Source: CAD feature listing. Evaluate the final solid. Frame: model axes, mm. A direction names the side the tool comes from. Give positions to 0.01 mm unless a question says otherwise; leave off trailing zeros. Order: outer loops, then holes, each group sorted by start corner. A loop starts at its lowest first (then second) coordinate and runs counter-clockwise, first axis right, second up. Notation, with made-up numbers: (45, -16) - (85, -16) arc R24 cw to (85, 13) - close; hole circle Ø8 at (-20.75, 74). An arc over 180 degrees is marked (long way). Use CSV: the item, a comma, the result in double quotes.
```python
from build123d import *

# Parameters (mm, degrees)
SKETCH1_W           = 12.7
SKETCH1_H           = 12.7
SKETCH1_W_2         = 9.525
SKETCH1_H_2         = 9.525
BOSS_EXTRUDE1_DEPTH = 254
CUT_EXTRUDE1_DEPTH  = 13.7
FILLET1_R           = 1.5875
CUT_EXTRUDE2_REACH  = 14.7
SKETCH3_R           = 2.032


with BuildPart() as part:
    # Sketch1 → Boss-Extrude1 (new body)
    with BuildSketch(Plane.XY):
        with Locations((6.35, 6.35)):
            Rectangle(SKETCH1_W, SKETCH1_H)
        with Locations((6.35, 6.35)):
            Rectangle(SKETCH1_W_2, SKETCH1_H_2, mode=Mode.SUBTRACT)
    extrude(amount=BOSS_EXTRUDE1_DEPTH)

    # Sketch2 → Cut-Extrude1 (cut, through all)
    with BuildSketch(Plane(origin=(0, 12.7, 0), x_dir=(1, 0, 0), z_dir=(0, 1, 0))):
        Polygon((0, -254), (12.7, -254), (12.7, -241.3), align=None)
        Polygon((0, 0), (12.7, -12.7), (12.7, 0), align=None)
    extrude(amount=-CUT_EXTRUDE1_DEPTH, mode=Mode.SUBTRACT)

    # Fillet1
    fillet1_edges = [part.edges().sort_by_distance(p)[0] for p in [
        (12.7, 12.7, 127),
        (12.7, 0, 127),
        (0, 12.7, 127),
        (0, 0, 127),
    ]]
    fillet(fillet1_edges, radius=FILLET1_R)

    # Sketch3 → Cut-Extrude2 (cut, up to next)
    with BuildSketch(Plane.ZY, mode=Mode.PRIVATE) as cut_extrude2_sk1:
        with Locations((136.525, 6.35)):
            Circle(SKETCH3_R)
    cut_extrude2_tool1 = extrude(cut_extrude2_sk1.sketch, amount=-CUT_EXTRUDE2_REACH, mode=Mode.PRIVATE) & part.part
    add(cut_extrude2_tool1.solids().sort_by_distance((0, 6.35, 136.525))[0], mode=Mode.SUBTRACT)
    # Sketch3 → Cut-Extrude2 (cut, up to next)
    with BuildSketch(Plane.ZY, mode=Mode.PRIVATE) as cut_extrude2_sk2:
        with Locations((117.475, 6.35)):
            Circle(SKETCH3_R)
    cut_extrude2_tool2 = extrude(cut_extrude2_sk2.sketch, amount=-CUT_EXTRUDE2_REACH, mode=Mode.PRIVATE) & part.part
    add(cut_extrude2_tool2.solids().sort_by_distance((0, 6.35, 117.475))[0], mode=Mode.SUBTRACT)


solid = part.part
```
Item 1: Set-up query: faces 5 (the flat face through (1.587, 6, 125)), 6 (the cylindrical face through (0.78, 5.57, 119.35)), 7 (the flat face through (6, 1, 6)). Return all of +Z, -Z, +X, -X, +Y, -Y with unobstructed straight access to the full face (end or side cutting, diameter ignored); none if empty.
Filled in:
face 5,"+Z, -Z"
face 6,"-X"
face 7,"-Z, +X, +Y, -Y"
Item 2: Section C-C on z = 141.5. Return the cut outline in (x, y) (1 decimal).
Filled in:
outline,"(0, 1.6) arc R1.6 ccw to (1.6, 0) - (11.1, 0) arc R1.6 ccw to (12.7, 1.6) - (12.7, 11.1) arc R1.6 ccw to (11.1, 12.7) - (1.6, 12.7) arc R1.6 ccw to (0, 11.1) - close; hole (1.6, 1.6) - (11.1, 1.6) - (11.1, 11.1) - (1.6, 11.1) - close"
Item 3: Material intervals for line 1 (X direction, y = 9.75, z = 209.5); line 2 (X direction, y = 11.25, z = 192), sorted ascending. Write a range as from..to.
Filled in:
line 1,"x = 0..1.59, 11.11..12.7"
line 2,"x = 0.01..12.69"
Item 4: First-contact query: pin 1 (3.5 mm diameter, centred on y = 6.35, z = 136.525, fed in from -X); pin 2 (5 mm diameter, centred on x = 9.5, y = 10, fed in from -Z); pin 3 (2 mm diameter, centred on x = 9.5, y = 10.5, fed in from -Z). Flat tips, straight axial feed; report the tip coordinate or a pass-through.
Filled in:
pin 1,"stops at x = 11.11"
pin 2,"stops at z = 7.26"
pin 3,"stops at z = 8.71"
Item 5: Mould query, pull axis Y, two halves, no side actions, for faces 1 (the flat face through (6, 12.7, 125)), 2 (the flat face through (11.112, 6, 125)), 3 (the cylindrical face through (0.783, 6.439, 134.495)), 4 (the flat face through (6, 1, 248)). Classes: released by +Y, released by -Y, zero draft, split by the parting line, or undercut.
Filled in:
face 1,"released by +Y"
face 2,"undercut"
face 3,"undercut"
face 4,"zero draft"
Item 6: Section A-A on y = 6.35. Return the cut outline in (x, z), then the cut area to 3 significant figures.
Filled in:
outline,"(0, 0) - (1.59, 1.59) - (1.59, 115.44) - (0, 115.44) - close; (0, 119.51) - (1.59, 119.51) - (1.59, 134.49) - (0, 134.49) - close; (0, 138.56) - (1.59, 138.56) - (1.59, 252.41) - (0, 254) - close; (11.11, 11.11) - (12.7, 12.7) - (12.7, 241.3) - (11.11, 242.89) - close"
area,"753 mm2"
Item 7: Section B-B on x = 4.5. Return the cut outline in (y, z), then the cut area to 3 significant figures.
Filled in:
outline,"(0, 4.5) - (1.59, 4.5) - (1.59, 249.5) - (0, 249.5) - close; (11.11, 4.5) - (12.7, 4.5) - (12.7, 249.5) - (11.11, 249.5) - close"
area,"778 mm2"
